Job drawing, mm, ordinate dimensions from the low corner. One solid piece. A direction names the side the tool comes from. Give positions to 0.01 mm unless a question says otherwise; leave off trailing zeros. Order: outer loops, then holes, each group sorted by start corner. A loop starts at its lowest first (then second) coordinate and runs counter-clockwise, first axis right, second up. Notation, with made-up numbers: M 55,-33.5 L 99,-33.5 A18 ccw 99,-7.5 Z; hole C 85.25,46.25 d2. An arc over 180 degrees is marked long. Use CSV: the item, a comma, the result in double quotes. Start each with the question number.
Item 1: Band-saw the part on D-D on z = 6.5. Write the cut outline in (x, y).
Item 2: Band-saw the part on A-A on x = 10. Write the cut outline in (y, z).
Item 3: Which spindle directions (+Z, -Z, +X, -X, +Y, -Y) get a long thin tool onto all of the face, cutting with end or side? Do the marked faces 1 and 2. Say none if no direction does.
Item 4: Pin check, flat tips, straight feed: P1, Ø5, axis at y = 10, z = 10, coming from the +X side; P2, Ø4, axis at x = 4, z = 12.5, coming from the +Y side. Stop position of each tip, or through.
Item 5: Band-saw the part on C-C on y = 11. Write the cut outline in (x, z).
Item 6: Band-saw the part on B-B on z = 10.75. Write the cut outline in (x, y) (1 decimal).
Item 7: Wall check: line 1 along Z through (x, y) = (10, 1.2). Give the ranges that are in metal, low to high.
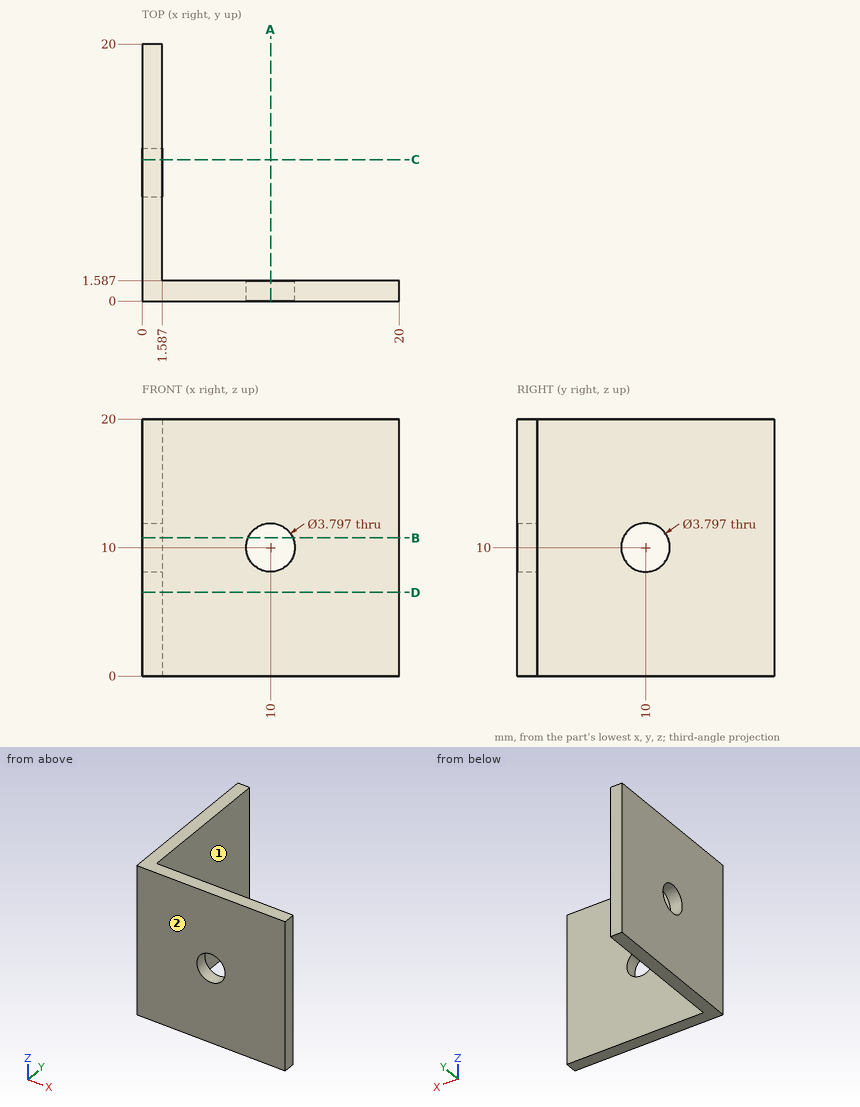
Model answer:
1,outline,"M 0,0 L 20,0 L 20,1.59 L 1.59,1.59 L 1.59,20 L 0,20 Z"
2,outline,"M 0,0 L 1.59,0 L 1.59,8.1 L 0,8.1 Z; M 0,11.9 L 1.59,11.9 L 1.59,20 L 0,20 Z"
3,face 1,"+Z, -Z, +X, +Y"
3,face 2,"+Z, -Z, +X, -X, -Y"
4,P1,"stops at x = 1.59"
4,P2,"stops at y = 1.59"
5,outline,"M 0,0 L 1.59,0 L 1.59,8.39 L 0,8.39 Z; M 0,11.61 L 1.59,11.61 L 1.59,20 L 0,20 Z"
6,outline,"M 0,0 L 8.3,0 L 8.3,1.6 L 1.6,1.6 L 1.6,8.3 L 0,8.3 Z; M 0,11.7 L 1.6,11.7 L 1.6,20 L 0,20 Z; M 11.7,0 L 20,0 L 20,1.6 L 11.7,1.6 Z"
7,line 1,"z = 0 to 8.1, 11.9 to 20"
